Part model, mm, in its own coordinate system. Give positions to 0.01 mm unless a question says otherwise; leave off trailing zeros. Order: outer loops, then holes, each group sorted by start corner. A loop starts at its lowest first (then second) coordinate and runs counter-clockwise, first axis right, second up. Notation, with made-up numbers: (32, -32) -> (68, -32) arc R13 cw to (68, -18) -> close; hole circle Ø4 at (26.5, 65.25). An arc over 180 degrees is marked (long way). Write item = value, one per line. Start each with the question number.
Item 1: Drill centre lines: line 1 along Y through (x, z) = (8, -1.3); line 2 along Y through (x, z) = (109, -0.05); line 3 along Y through (x, z) = (7.5, -1.8). Where is each one in solid material? Low to high.
Item 2: Band-saw the part on A-A on x = 83. Write the cut outline in (y, z).
Item 3: Pull direction Y, two halves, no side cores. Call faces 1 (the face through (7.67, 110.48, -0.99)), 2 (the face through (53, 55, 0)), 3 (the face through (76, 74, -1)), 4 (the face through (7.67, 85.48, -0.99)): +Y half, -Y half, draft (parallel to the pull), parting line (faces both ways), or undercut.
Item 4: Band-saw the part on C-C on z = -0.9. Count the separate pieces of the cut face and the enclosed holes in it, plus the area to 3 significant figures.
Item 5: Band-saw the part on D-D on y = 8. Write the cut outline in (x, z).
Item 6: Flat gauge pin, fed straight in: P1, Ø4.5, axis at x = 83, y = 8, coming from the +Z side. Where does the tip first touch, or does it go through?
```python
from build123d import *

# Parameters (mm, degrees)
SM_BASE_FLANGE_1_DEPTH = 2
SKETCH_7_R             = 5.5
SKETCH_7_R_2           = 2.5
CUT_EXTRUDE_1_DEPTH    = 10


# Sheet-metal steps are written as plain solids
with BuildPart() as part:
    # Sketch 1 → Базовая кромка1 (new body)
    with BuildSketch(Plane.XY):
        Polygon((0, 0), (140, 0), (140, 10), (10, 140), (0, 140), align=None)
    extrude(amount=-SM_BASE_FLANGE_1_DEPTH)

    # Эскиз7 → Вырез-Вытянуть1 (cut)
    with BuildSketch(Plane.XY):
        Polygon((10, 0), (0, 10), (0, 0), align=None)
        with Locations((11, 11)):
            Circle(SKETCH_7_R)
        with Locations((8, 33)):
            Circle(SKETCH_7_R_2)
        with Locations((33, 8)):
            Circle(SKETCH_7_R_2)
        with Locations((58, 8)):
            Circle(SKETCH_7_R_2)
        with Locations((83, 8)):
            Circle(SKETCH_7_R_2)
        with Locations((8, 58)):
            Circle(SKETCH_7_R_2)
        with Locations((8, 108)):
            Circle(SKETCH_7_R_2)
        with Locations((8, 83)):
            Circle(SKETCH_7_R_2)
        with Locations((108, 8)):
            Circle(SKETCH_7_R_2)
    extrude(amount=-CUT_EXTRUDE_1_DEPTH, mode=Mode.SUBTRACT)


solid = part.part
```
Values found:
q1.line_1 = 2 to 6.39, 15.61 to 30.5, 35.5 to 55.5, 60.5 to 80.5, 85.5 to 105.5, 110.5 to 140
q1.line_2 = 0 to 5.71, 10.29 to 41
q1.line_3 = 2.5 to 6.76, 15.24 to 30.55, 35.45 to 55.55, 60.45 to 80.55, 85.45 to 105.55, 110.45 to 140
q2.outline = (0, -2) -> (5.5, -2) -> (5.5, 0) -> (0, 0) -> close; (10.5, -2) -> (67, -2) -> (67, 0) -> (10.5, 0) -> close
q3.face_1 = undercut
q3.face_2 = draft
q3.face_3 = +Y half
q3.face_4 = undercut
q4.separate_pieces = 1
q4.enclosed_holes = 9
q4.area = 10,800 mm^2
q5.outline = (2, -2) -> (6.39, -2) -> (6.39, 0) -> (2, 0) -> close; (15.61, -2) -> (30.5, -2) -> (30.5, 0) -> (15.61, 0) -> close; (35.5, -2) -> (55.5, -2) -> (55.5, 0) -> (35.5, 0) -> close; (60.5, -2) -> (80.5, -2) -> (80.5, 0) -> (60.5, 0) -> close; (85.5, -2) -> (105.5, -2) -> (105.5, 0) -> (85.5, 0) -> close; (110.5, -2) -> (140, -2) -> (140, 0) -> (110.5, 0) -> close
q6.P1 = through
